from build123d import *

# Parameters (mm, degrees)
SKETCH_1_R          = 3.35
EXTRUDE_1_DEPTH     = 7
SKETCH_2_W          = 11
SKETCH_2_H          = 20
EXTRUDE_2_DEPTH     = 5
FILLET_1_R          = 5
FILLET_2_R          = 1
FILLET_4_R          = 1
FILLET_11_R         = 6
SKETCH_3_R          = 2
CUT_EXTRUDE_2_DEPTH = 10


with BuildPart() as part:
    # Эскиз1 → Бобышка-Вытянуть1 (new body)
    with BuildSketch(Plane.XY):
        Polygon((-5, 10), (6, 10), (6, -10), (-5, -7), align=None)
        Circle(SKETCH_1_R, mode=Mode.SUBTRACT)
    extrude(amount=EXTRUDE_1_DEPTH)

    # Эскиз2 → Бобышка-Вытянуть2 (add)
    with BuildSketch(Plane(origin=(0, 10, 0), x_dir=(1, 0, 0), z_dir=(0, 1, 0))):
        with Locations((0.5, 3)):
            Rectangle(SKETCH_2_W, SKETCH_2_H)
    extrude(amount=EXTRUDE_2_DEPTH)

    # Скругление1
    fillet_1_edges = [part.edges().sort_by_distance(p)[0] for p in [
        (0.5, 10, 0),
    ]]
    fillet(fillet_1_edges, radius=FILLET_1_R)

    # Скругление2
    fillet_2_edges = [part.edges().sort_by_distance(p)[0] for p in [
        (-3.35, 0, 0),
    ]]
    fillet(fillet_2_edges, radius=FILLET_2_R)

    # Скругление4
    fillet_4_edges = [part.edges().sort_by_distance(p)[0] for p in [
        (0.5, 15, 7),
    ]]
    fillet(fillet_4_edges, radius=FILLET_4_R)

    # Скругление11
    # the kernel refuses this fillet: 6 mm, written as the material it takes off along each edge
    with BuildSketch(Plane(origin=(6, -5, -13), x_dir=(0, 0, 1), z_dir=(0, 1, 0)), Plane(origin=(-5, -5, -13), x_dir=(1, 0, 0), z_dir=(0, 1, 0))) as fillet_11_piece_1:
        with BuildLine():
            CenterArc((FILLET_11_R, -FILLET_11_R), FILLET_11_R, 90, 90)
            Line((0, -FILLET_11_R), (0, 0))
            Line((0, 0), (FILLET_11_R, 0))
        make_face()
    extrude(amount=35, mode=Mode.SUBTRACT)

    # Эскиз3 → Вырез-Вытянуть2 (cut)
    with BuildSketch(Plane.XZ.offset(-10)):
        with Locations(Location((0.5, -9, 0), (0, 0, 270))):
            Circle(SKETCH_3_R)
    extrude(amount=-CUT_EXTRUDE_2_DEPTH, mode=Mode.SUBTRACT)


solid = part.part
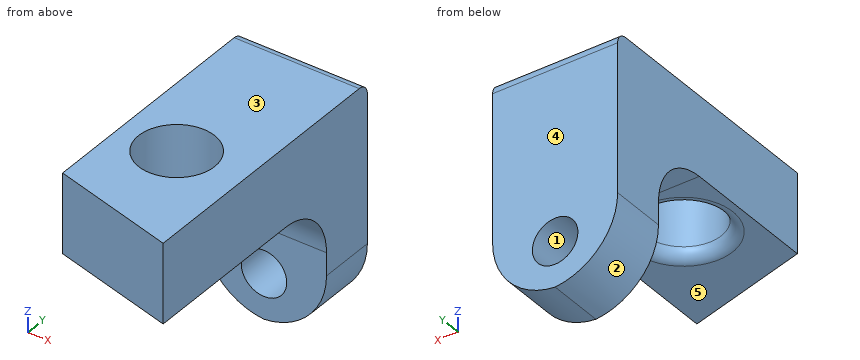
Source: CAD feature listing. Evaluate the final solid. Frame: model axes, mm. Face numbers are marked on the shaded views. A direction names the side the tool comes from. Give positions to 0.01 mm unless a question says otherwise; leave off trailing zeros. Write each loop counter-clockwise with the first axis right and the second up, starting at its lowest first coordinate (ties: lowest second). Pieces come first, ordered by that corner, then holes. Notation, with made-up numbers: M 71,-34.75 L 115,-34.75 A8 ccw 115,-28.75 Z; hole C 68.5,79.5 d6. An arc over 180 degrees is marked long. Answer as a JSON object with one key per item and string values.
Q1. Mould query, pull axis X, two halves, no side actions, for the marked faces 1, 2 and 3. Classes: +X half, -X half, draft (parallel to the pull), parting line (faces both ways), or undercut.
Geometry check:
{"face 1": "undercut", "face 2": "-X half", "face 3": "draft"}
Q2. Contact query for flat-ended pins moving along their axis: P1, Ø3, axis at x = 0, y = 9, coming from the -Z side; P2, Ø3, axis at y = 11.5, z = -9.5, coming from the +X side; P3, Ø5.5, axis at x = -1.5, y = -6, coming from the -Z side; P4, Ø2, axis at x = -3, z = 4, coming from the -Y side. Output: stop coordinate, or through.
Geometry check:
{"P1": "stops at z = -12.98", "P2": "stops at x = 5.92", "P3": "stops at z = 0", "P4": "stops at y = -7.82"}
Q3. Access query for the marked faces 4 and 5. Directions: +Z, -Z, +X, -X, +Y, -Y. A direction counts if a zero-diameter tool reaches every point of the face in a straight line with its end or side. Return the directions, or none.
Geometry check:
{"face 4": "+Z, -Z, +X, -X, +Y", "face 5": "-Z, +X, -X, -Y"}
Q4. Cut plane A-A, the plane y = 0. Return the cut outline in (x, z), then the cut area to 3 significant figures.
Geometry check:
{"outline": "M -5,0 L -4.35,0 A1 ccw -3.35,1 L -3.35,7 L -5,7 Z; M 3.35,1 A1 ccw 4.35,0 L 6,0 L 6,7 L 3.35,7 Z", "area": "29.7 mm^2"}
Q5. Cut plane D-D, the plane z = -6. Return the cut outline in (x, y), then the cut area to 3 significant figures.
Geometry check:
{"outline": "M -5,10 L 6,10 L 6,15 L -5,15 Z", "area": "55.0 mm^2"}
Q6. Cut plane C-C, the plane x = 0. Return the cut outline in (y, z), then the cut area to 3 significant figures.
Geometry check:
{"outline": "M -8.36,0 L -4.35,0 A1 ccw -3.35,1 L -3.35,7 L -8.36,7 Z; M 3.35,1 A1 ccw 4.35,0 L 5,0 A5 cw 10,-5 L 10,-7.06 L 15,-7.06 L 15,6 A1 ccw 14,7 L 3.35,7 Z; M 10,-12.92 L 15,-12.92 L 15,-10.94 L 10,-10.94 Z", "area": "167 mm^2"}
Q7. Cut plane B-B, the plane z = -9. Return the cut outline in (x, y).
Geometry check:
{"outline": "M -4.66,10 L -1.5,10 L -1.5,15 L -4.66,15 Z; M 2.5,10 L 5.66,10 L 5.66,15 L 2.5,15 Z"}
Q8. Ray query, line 1 along Z through (x, y) = (4, -7.5); line 2 along Y through (x, z) = (4.5, -7.5); line 3 along Z through (x, y) = (0.75, 11.5). Return the intervals inside material, ascending.
Geometry check:
{"line 1": "z = 0 to 7", "line 2": "y = 10 to 15", "line 3": "z = -12.95 to -10.98, -7.02 to 7"}
